Verification items for the finished model (mm, model axes). A direction names the side the tool comes from. Round coordinates to 2 decimals unless told otherwise and drop trailing zeros. Order: outer loops, then holes, each group sorted by start corner. A loop starts at its lowest first (then second) coordinate and runs counter-clockwise, first axis right, second up. Notation, with made-up numbers: M 64,68 L 77,68 A15 ccw 77,89 Z; hole C -34.5,64.25 d11. An arc over 180 degrees is marked long. Use one line per item in the form item = value. Start each with the question number.
Item 1: Thickness scan on probe 1 along Z at (x, y) = (-18.5, 3) (3 decimals); probe 2 along Y at (x, z) = (-27.5, 46.5) (3 decimals); probe 3 along X at (y, z) = (-5, 71). Record the ranges inside material, lowest first. Write a range as [from, to].
Item 2: Tool access check on faces 4 (the cylindrical face through (24.405, 23.69, 0.751)), 5 (the cylindrical face through (34.16, -20.41, 39.4)), 6 (the cylindrical face through (34.16, 20.41, 39.98)). Record the directions out of +Z, -Z, +X, -X, +Y, -Y that give a thin tool (end or side, any length) a straight path to the whole face; none if there is none.
Item 3: Release check for a two-part mould opening along X. For faces 1 (the cylindrical face through (-34.26, 0.22, 14.61)), 2 (the flat face through (-22, 0, 1.524)), 3 (the cylindrical face through (21.06, 27.11, 0.75)) record: +X half, -X half, draft (parallel to the pull), parting line (faces both ways), or undercut.
Item 4: Cross-section at D-D on x = -24. Enter the section's corners in (y, z) (3 decimals).
Item 5: Cross-section at B-B on z = 51. Enter the section's corners in (x, y) (3 decimals).
Item 6: Cross-section at A-A on x = 16. Enter the section's corners in (y, z) (3 decimals), then the cut area to 3 significant figures.
Item 7: Go/stop test with flat-tipped pins: pin 1 Ø1.5 at (x, z) = (-13.5, 60.5) entering from -Y (3 decimals); pin 2 Ø5.5 at (x, y) = (-20.5, 13.5) entering from +Z (3 decimals); pin 3 Ø3 at (y, z) = (-18.5, 17.5) entering from +X. Record where each tip stops, or that it passes through.
Item 8: Cross-section at C-C on y = 5. Enter the section's corners in (x, z) (3 decimals), then the cut area to 3 significant figures.
from build123d import *

# Parameters (mm, degrees)
F0_W             = 12.7
F0_H             = 74.676
F0_W_2           = 19.05
F0_H_2           = 1.524
F1_DEPTH         = 31.75
F3_W             = 44.45
F3_H             = 53.975
F4_DEPTH         = 36.068
F6_DEPTH         = 1.524
F6_COPIES2_COUNT = 2
F6_COPIES2_PITCH = 68.174755
F7_R             = 6.35
F8_R             = 6.35


# Not quite as in the source:
# - a pattern or mirror of a feature is missing from the dataset's text; its kind, count and spacing are read off the source's solid


with BuildPart() as f1:
    # F0 (on Front) → F1 (new body, symmetric)
    with BuildSketch(Plane.XZ):
        with Locations((-6.35, 38.862)):
            Rectangle(F0_W, F0_H)
        with Locations((-22.225, 0.762)):
            Rectangle(F0_W_2, F0_H_2)
        with Locations((-6.35, 0.762)):
            Rectangle(F0_W, F0_H_2)
    extrude(amount=F1_DEPTH, both=True)

    # F2: F1 across plane


with BuildPart() as f1_1:
    add(f1.part)
    add(f1.part.mirror(Plane.YZ))

    # F3 (on Right) → F4 (join, symmetric)
    with BuildSketch(Plane.YZ):
        with Locations((0, 39.6875)):
            Rectangle(F3_W, F3_H)
    extrude(amount=F4_DEPTH, both=True)

    # F5 (on face) → F6 (cut, through all)
    with BuildSketch(Plane(origin=(0, 0, 0), x_dir=(1, 0, 0), z_dir=(0, 0, -1))):
        with BuildLine():
            Line((22.72538, 23.0116418839), (22.74062, 23.0116418839))
            ThreePointArc((22.74062, 23.0116418839), (24.4235199971, 23.7087218868), (25.1206, 25.3916218839))
            Line((25.1206, 25.3916218839), (25.1206, 25.4083781161))
            ThreePointArc((25.1206, 25.4083781161), (24.4235199971, 27.0912781132), (22.74062, 27.7883581161))
            Line((22.74062, 27.7883581161), (22.72538, 27.7883581161))
            ThreePointArc((22.72538, 27.7883581161), (21.0424800029, 27.0912781132), (20.3454, 25.4083781161))
            Line((20.3454, 25.4083781161), (20.3454, 25.3916218839))
            ThreePointArc((20.3454, 25.3916218839), (21.0424800029, 23.7087218868), (22.72538, 23.0116418839))
        make_face()
    f6 = extrude(amount=-F6_DEPTH, mode=Mode.SUBTRACT)

    # F6_copies: F6 across plane
    add(f6.mirror(Plane.ZX), mode=Mode.SUBTRACT)

    # F6_copies1: F6 across plane
    add(f6.mirror(Plane(origin=(0, 0, 0), x_dir=(0, 0, -1), z_dir=(-1, 0, 0))), mode=Mode.SUBTRACT)

    # F6_copies2: F6 ×2
    with Locations(*[Vector(-0.666903758, 0.7451438637, 0) * (i * F6_COPIES2_PITCH) for i in range(1, F6_COPIES2_COUNT)]):
        add(f6, mode=Mode.SUBTRACT)

    # F7
    f7_edges = [f1_1.edges().sort_by_distance(p)[0] for p in [
        (24.384, -22.225, 66.675),
        (24.384, 22.225, 66.675),
        (24.384, 22.225, 12.7),
        (24.384, -22.225, 12.7),
        (-24.384, -22.225, 12.7),
        (-24.384, -22.225, 66.675),
        (-24.384, 22.225, 66.675),
        (-24.384, 22.225, 12.7),
    ]]
    fillet(f7_edges, radius=F7_R)

    # F8
    f8_edges = [f1_1.edges().sort_by_distance(p)[0] for p in [
        (-36.068, 22.225, 39.6875),
        (-36.068, 20.365128, 14.559872),
        (-36.068, 20.365128, 64.815128),
        (-36.068, 0, 12.7),
        (-36.068, 0, 66.675),
        (-36.068, -20.365128, 14.559872),
        (-36.068, -20.365128, 64.815128),
        (-36.068, -22.225, 39.6875),
        (36.068, 22.225, 39.6875),
        (36.068, 20.365128, 14.559872),
        (36.068, 20.365128, 64.815128),
        (36.068, 0, 12.7),
        (36.068, 0, 66.675),
        (36.068, -20.365128, 14.559872),
        (36.068, -20.365128, 64.815128),
        (36.068, -22.225, 39.6875),
    ]]
    fillet(f8_edges, radius=F8_R)


solid = f1_1.part
Output values:
q1.probe_1 = [0, 1.524], [12.7, 66.675]
q1.probe_2 = [-22.225, 22.225]
q1.probe_3 = [-12.7, 12.7]
q2.face_4 = +Z, -Z
q2.face_5 = +Z, +X, -Y
q2.face_6 = +Z, +X, +Y
q3.face_1 = -X half
q3.face_2 = draft
q3.face_3 = undercut
q4.outline = M -31.75,0 L -27.428,0 L -27.428,1.524 L -31.75,1.524 Z; M -23.372,0 L 23.372,0 L 23.372,1.524 L -23.372,1.524 Z; M -22.225,19.05 A6.35 ccw -15.875,12.7 L 15.875,12.7 A6.35 ccw 22.225,19.05 L 22.225,60.325 A6.35 ccw 15.875,66.675 L -15.875,66.675 A6.35 ccw -22.225,60.325 Z; M 27.428,0 L 31.75,0 L 31.75,1.524 L 27.428,1.524 Z
q5.outline = M -36.068,-15.875 A6.35 ccw -29.718,-22.225 L -12.7,-22.225 L -12.7,-31.75 L 12.7,-31.75 L 12.7,-22.225 L 29.718,-22.225 A6.35 ccw 36.068,-15.875 L 36.068,15.875 A6.35 ccw 29.718,22.225 L 12.7,22.225 L 12.7,31.75 L -12.7,31.75 L -12.7,22.225 L -29.718,22.225 A6.35 ccw -36.068,15.875 Z
q6.outline = M -31.75,0 L 31.75,0 L 31.75,1.524 L -31.75,1.524 Z; M -22.225,19.05 A6.35 ccw -15.875,12.7 L 15.875,12.7 A6.35 ccw 22.225,19.05 L 22.225,60.325 A6.35 ccw 15.875,66.675 L -15.875,66.675 A6.35 ccw -22.225,60.325 Z
q6.area = 2,460 mm2
q7.pin_1 = -22.225
q7.pin_2 = 66.675
q7.pin_3 = 35.88
q8.outline = M -36.068,19.05 A6.35 ccw -29.718,12.7 L -12.7,12.7 L -12.7,1.524 L -31.75,1.524 L -31.75,0 L 31.75,0 L 31.75,1.524 L 12.7,1.524 L 12.7,12.7 L 29.718,12.7 A6.35 ccw 36.068,19.05 L 36.068,60.325 A6.35 ccw 29.718,66.675 L 12.7,66.675 L 12.7,76.2 L -12.7,76.2 L -12.7,66.675 L -29.718,66.675 A6.35 ccw -36.068,60.325 Z
q8.area = 4,480 mm2
